```python
from build123d import *

# Parameters (mm, degrees)
BOSS_EXTRUDE1_START = -2.3
SKETCH2_R           = 4
SKETCH2_R_2         = 2.6
BOSS_EXTRUDE1_DEPTH = 1.8
CHAMFER1_SIZE       = 0.5
SKETCH3_W           = 0.5
SKETCH3_H           = 2
SKETCH3_W_2         = 2.2
SKETCH3_H_2         = 0.5
SKETCH3_W_3         = 0.638814793
BOSS_EXTRUDE2_DEPTH = 3
SKETCH4_W           = 2.2
SKETCH4_H           = 0.5
BOSS_EXTRUDE3_DEPTH = 3.3


with BuildPart() as part:
    # Sketch1 → Revolve1 (revolve)
    with BuildSketch(Plane(origin=(0, 0, 0), x_dir=(0, 0, -1), z_dir=(1, 0, 0)), mode=Mode.PRIVATE) as revolve1_sk:
        Polygon((0, 1.75), (0, 2.2), (0.8, 3), (4.5, 3), (4.5, 4), (16.2, 4), (16.2, 0), (13.508423887, 0), (13.508423887, 1.75), align=None)
    revolve(revolve1_sk.sketch.rotate(Axis((0, 0, 3.985074627), (0, 0, -1)), 90), axis=Axis((0, 0, 3.985074627), (0, 0, -1)))

    # Sketch2 → Boss-Extrude1 (add)
    with BuildSketch(Plane.XY.offset(BOSS_EXTRUDE1_START)):
        Circle(SKETCH2_R)
        Circle(SKETCH2_R_2, mode=Mode.SUBTRACT)
    extrude(amount=BOSS_EXTRUDE1_DEPTH)

    # Chamfer1
    chamfer1_edges = [part.edges().sort_by_distance(p)[0] for p in [
        (-4, 0, -0.5),
    ]]
    chamfer(chamfer1_edges, length=CHAMFER1_SIZE)

    # Sketch3 → Boss-Extrude2 (add)
    with BuildSketch(Plane(origin=(0, 0, -16.2), x_dir=(-1, 0, 0), z_dir=(0, 0, -1))):
        with Locations((-2.993209108, 0)):
            Rectangle(SKETCH3_W, SKETCH3_H)
        with Locations((0, 2.862816669)):
            Rectangle(SKETCH3_W_2, SKETCH3_H_2)
        with Locations((2.993209109, 0)):
            Rectangle(SKETCH3_W_3, SKETCH3_H)
    extrude(amount=BOSS_EXTRUDE2_DEPTH)

    # Sketch4 → Boss-Extrude3 (add)
    with BuildSketch(Plane(origin=(0, 0, -19.2), x_dir=(-1, 0, 0), z_dir=(0, 0, -1))):
        with Locations((0, 2.862816669)):
            Rectangle(SKETCH4_W, SKETCH4_H)
    extrude(amount=BOSS_EXTRUDE3_DEPTH)


solid = part.part
```
Input: part model. Units: mm. Frame: model coordinates. A direction names the side the tool comes from. Give positions to 0.01 mm unless a question says otherwise; leave off trailing zeros. Order: outer loops, then holes, each group sorted by start corner. A loop starts at its lowest first (then second) coordinate and runs counter-clockwise, first axis right, second up.
1. Mould query, pull axis Y, two halves, no side actions, for faces 4 (the flat face through (1, 3, -2.3)), 5 (the cylindrical face through (0.81, 1.55, -6.66)), 6 (the flat face through (0, 0, -13.508)), 7 (the flat face through (0, 2.613, -19)). Classes: released by +Y, released by -Y, zero draft, split by the parting line, or undercut.
Derived:
face 4: zero draft
face 5: undercut
face 6: undercut
face 7: released by -Y
2. Section A-A on x = 0. Return the cut outline in (y, z), and give its area (3 significant figures).
Derived:
outline: (-4, -16.2) - (2.61, -16.2) - (2.61, -22.5) - (3.11, -22.5) - (3.11, -16.2) - (4, -16.2) - (4, -4.5) - (3, -4.5) - (3, -2.3) - (4, -2.3) - (4, -1) - (3.5, -0.5) - (2.7, -0.5) - (2.2, 0) - (1.75, 0) - (1.75, -13.51) - (-1.75, -13.51) - (-1.75, 0) - (-2.2, 0) - (-2.7, -0.5) - (-3.5, -0.5) - (-4, -1) - (-4, -2.3) - (-3, -2.3) - (-3, -4.5) - (-4, -4.5) - close
area: 79.3 mm2
3. Section C-C on z = -11.25. Return the cut outline in (x, y).
Derived:
outline: circle Ø8 at (0, 0); hole circle Ø3.5 at (0, 0)
4. Pin query (flat end, axial travel): pin 1 (1.1 mm diameter, centred on x = 0, z = -18.5, fed in from -Y); pin 2 (1.6 mm diameter, centred on y = 0, z = -18, fed in from -X); pin 3 (1 mm diameter, centred on y = 2, z = -9.5, fed in from -X). Return the tip coordinate at first contact, or that it passes through.
Derived:
pin 1: stops at y = 2.61
pin 2: stops at x = -3.31
pin 3: stops at x = -3.71
5. Material intervals for L1, parallel to Z at x = -2.5, y = 2; L2, parallel to Y at x = 0, z = -6.5; L3, parallel to Y at x = 0, z = -3, sorted ascending.
Derived:
L1: z = -16.2 to -4.5, -2.3 to -0.5
L2: y = -4 to -1.75, 1.75 to 4
L3: y = -3 to -1.75, 1.75 to 3
6. Section D-D on z = -19.75. Return the cut outline in (x, y).
Derived:
outline: (-1.1, 2.61) - (1.1, 2.61) - (1.1, 3.11) - (-1.1, 3.11) - close
7. Reachability of faces 1 (the flat face through (1, -3, -0.5)), 2 (the cylindrical face through (2.86, -0.9, -3.42)), 3 (the flat face through (-2.674, 0, -18)) from +Z, -Z, +X, -X, +Y, -Y: full face, straight path, thin tool, end or side. Return the list, or none.
Derived:
face 1: +Z
face 2: none
face 3: -Z, +Y, -Y
